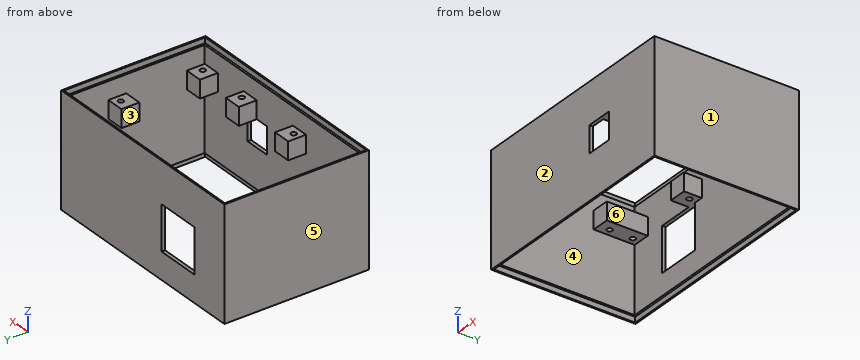
```python
from build123d import *

# Parameters (mm, degrees)
F0_W      = 124.8
F0_H      = 81
F1_DEPTH  = 63
F2_W      = 123.1
F2_H      = 79.3
F3_DEPTH  = 3
F4_W      = 123.1
F4_H      = 79.3
F5_DEPTH  = 3
F6_W      = 120.8
F6_H      = 77
F7_DEPTH  = 60.001
F8_W      = 21
F8_H      = 10
F9_DEPTH  = 10
F10_W     = 23
F10_H     = 10
F11_DEPTH = 10
F12_W     = 10
F12_H     = 10
F13_DEPTH = 10
F14_W     = 10
F14_H     = 10
F15_DEPTH = 10
F16_W     = 10
F16_H     = 10
F17_DEPTH = 10
F18_W     = 10
F18_H     = 10
F19_DEPTH = 10
F20_W     = 10
F20_H     = 10
F21_DEPTH = 10
F22_R     = 1.5
F23_DEPTH = 50.001
F24_R     = 1.5
F25_DEPTH = 50.001
F26_R     = 1.5
F27_DEPTH = 50.001
F28_R     = 1.5
F29_DEPTH = 50.001
F30_R     = 1.5
F31_DEPTH = 50.001
F32_R     = 1.5
F33_DEPTH = 50.001
F34_R     = 1.5
F35_DEPTH = 50.001
F36_R     = 1.5
F37_DEPTH = 50.001
F38_R     = 1.5
F39_DEPTH = 50.001
F40_W     = 25
F40_H     = 25
F41_DEPTH = 2.001
F42_W     = 15
F42_H     = 15
F43_DEPTH = 12


with BuildPart() as f1:
    # F0 (on Top) → F1 (new body)
    with BuildSketch(Plane.XY):
        Rectangle(F0_W, F0_H)
    extrude(amount=F1_DEPTH)

    # F2 (on face) → F3 (cut)
    with BuildSketch(Plane(origin=(0, 0, 0), x_dir=(1, 0, 0), z_dir=(0, 0, -1))):
        Rectangle(F2_W, F2_H)
    extrude(amount=-F3_DEPTH, mode=Mode.SUBTRACT)

    # F4 (on face) → F5 (cut)
    with BuildSketch(Plane.XY.offset(63)):
        Rectangle(F4_W, F4_H)
    extrude(amount=-F5_DEPTH, mode=Mode.SUBTRACT)

    # F6 (on face) → F7 (cut, through all)
    with BuildSketch(Plane.XY.offset(60)):
        Rectangle(F6_W, F6_H)
    extrude(amount=-F7_DEPTH, mode=Mode.SUBTRACT)

    # F8 (on face) → F9 (join)
    with BuildSketch(Plane.YZ.offset(-60.4)):
        with Locations((-28, 45)):
            Rectangle(F8_W, F8_H)
    extrude(amount=F9_DEPTH)

    # F10 (on face) → F11 (join)
    with BuildSketch(Plane.YZ.offset(-60.4)):
        with Locations((27, 45)):
            Rectangle(F10_W, F10_H)
    extrude(amount=F11_DEPTH)

    # F12 (on face) → F13 (join)
    with BuildSketch(Plane(origin=(60.4, 0, 0), x_dir=(0, -1, 0), z_dir=(-1, 0, 0))):
        with Locations((33.5, 45)):
            Rectangle(F12_W, F12_H)
    extrude(amount=F13_DEPTH)

    # F14 (on face) → F15 (join)
    with BuildSketch(Plane(origin=(60.4, 0, 0), x_dir=(0, -1, 0), z_dir=(-1, 0, 0))):
        with Locations((-10.5, 45)):
            Rectangle(F14_W, F14_H)
    extrude(amount=F15_DEPTH)

    # F16 (on face) → F17 (join)
    with BuildSketch(Plane(origin=(0, -38.5, 0), x_dir=(-1, 0, 0), z_dir=(0, 1, 0))):
        with Locations((-25.6, 45)):
            Rectangle(F16_W, F16_H)
    extrude(amount=F17_DEPTH)

    # F18 (on face) → F19 (join)
    with BuildSketch(Plane(origin=(0, -38.5, 0), x_dir=(-1, 0, 0), z_dir=(0, 1, 0))):
        with Locations((12.1, 45)):
            Rectangle(F18_W, F18_H)
    extrude(amount=F19_DEPTH)

    # F20 (on face) → F21 (join)
    with BuildSketch(Plane.XZ.offset(-38.5)):
        with Locations((-14.06, 45)):
            Rectangle(F20_W, F20_H)
    extrude(amount=F21_DEPTH)

    # F22 (on face) → F23 (cut, through all)
    with BuildSketch(Plane.XY.offset(50)):
        with Locations((-56.4, -34.5)):
            Circle(F22_R)
    extrude(amount=-F23_DEPTH, mode=Mode.SUBTRACT)

    # F24 (on face) → F25 (cut, through all)
    with BuildSketch(Plane.XY.offset(50)):
        with Locations((-56.4, -23.5)):
            Circle(F24_R)
    extrude(amount=-F25_DEPTH, mode=Mode.SUBTRACT)

    # F26 (on face) → F27 (cut, through all)
    with BuildSketch(Plane.XY.offset(50)):
        with Locations((-56.4, 34.5)):
            Circle(F26_R)
    extrude(amount=-F27_DEPTH, mode=Mode.SUBTRACT)

    # F28 (on face) → F29 (cut, through all)
    with BuildSketch(Plane.XY.offset(50)):
        with Locations((-56.4, 21.5)):
            Circle(F28_R)
    extrude(amount=-F29_DEPTH, mode=Mode.SUBTRACT)

    # F30 (on face) → F31 (cut, through all)
    with BuildSketch(Plane.XY.offset(50)):
        with Locations((56.4, -34.5)):
            Circle(F30_R)
    extrude(amount=-F31_DEPTH, mode=Mode.SUBTRACT)

    # F32 (on face) → F33 (cut, through all)
    with BuildSketch(Plane.XY.offset(50)):
        with Locations((56.4, 11.5)):
            Circle(F32_R)
    extrude(amount=-F33_DEPTH, mode=Mode.SUBTRACT)

    # F34 (on face) → F35 (cut, through all)
    with BuildSketch(Plane.XY.offset(50)):
        with Locations((26.6, -34.5)):
            Circle(F34_R)
    extrude(amount=-F35_DEPTH, mode=Mode.SUBTRACT)

    # F36 (on face) → F37 (cut, through all)
    with BuildSketch(Plane.XY.offset(50)):
        with Locations((-13.1, -34.5)):
            Circle(F36_R)
    extrude(amount=-F37_DEPTH, mode=Mode.SUBTRACT)

    # F38 (on face) → F39 (cut, through all)
    with BuildSketch(Plane.XY.offset(50)):
        with Locations((-13.06, 34.5)):
            Circle(F38_R)
    extrude(amount=-F39_DEPTH, mode=Mode.SUBTRACT)

    # F40 (on face) → F41 (cut, through all)
    with BuildSketch(Plane.XZ.offset(-38.5)):
        with Locations((-26.9, 27.5)):
            Rectangle(F40_W, F40_H)
    extrude(amount=-F41_DEPTH, mode=Mode.SUBTRACT)

    # F42 (on face) → F43 (cut)
    with BuildSketch(Plane.XZ.offset(40.5)):
        with Locations((20.1, 32.5)):
            Rectangle(F42_W, F42_H)
    extrude(amount=-F43_DEPTH, mode=Mode.SUBTRACT)


solid = f1.part
```
Work out the finished part from the listing and answer in its coordinate system (mm). Face numbers are marked on the shaded views. A direction names the side the tool comes from. Give positions to 0.01 mm unless a question says otherwise; leave off trailing zeros. Loops run counter-clockwise (first coordinate to the right, second up) from the corner with the lowest first, then second, coordinate; pieces in that order, holes last. Notation, with made-up numbers: M 43.5,56 L 85.5,56 A19 ccw 85.5,74 Z; hole C 66,84 d7. An arc over 180 degrees is marked long. One line per item, written item: value. Start each with the question number.
1. Determine the mould class of the marked faces 1, 2 and 3 for opening direction Y: released by +Y, released by -Y, zero draft, split by the parting line, or undercut.
2. Find section D-D (x = 11). Give the vertices of the cut face in (y, z).
3. Which of the six approach directions +Z, -Z, +X, -X, +Y, -Y give full straight-line access (tool end or side, diameter ignored) to the marked faces 4, 5 and 6?
4. Find section C-C (x = -30). Give the vertices of the cut face in (y, z).
5. Each of these flat-tipped pins is pushed along its axis until it touches: P1, Ø10, axis at x = 25.5, y = -29, coming from the +Z side; P2, Ø4, axis at x = 56.4, y = -34.5, coming from the -Z side. Where does it stop, or does it pass through?
6. Find section B-B (z = 33.5). Give the vertices of the cut face in (x, y), and give its area (3 significant figures).
7. Find section A-A (y = -23.5). Give the vertices of the cut face in (x, z).
8. Find the intervals of material crossed by probe 1 along Y at (x, z) = (56.4, 45.5); probe 2 along Y at (x, z) = (-56.4, 42.75); probe 3 along Y at (x, z) = (-13.06, 43.75), in increasing order.
Reported:
1. face 1: zero draft
1. face 2: released by -Y
1. face 3: undercut
2. outline: M -40.5,0 L -39.65,0 L -39.65,3 L -38.5,3 L -38.5,60 L -39.65,60 L -39.65,63 L -40.5,63 Z; M 38.5,3 L 39.65,3 L 39.65,0 L 40.5,0 L 40.5,63 L 39.65,63 L 39.65,60 L 38.5,60 Z
3. face 4: none
3. face 5: +Z, -Z, -X, +Y, -Y
3. face 6: +Z, -Z
4. outline: M -40.5,0 L -39.65,0 L -39.65,3 L -38.5,3 L -38.5,60 L -39.65,60 L -39.65,63 L -40.5,63 Z; M 38.5,3 L 39.65,3 L 39.65,0 L 40.5,0 L 40.5,15 L 38.5,15 Z; M 38.5,40 L 40.5,40 L 40.5,63 L 39.65,63 L 39.65,60 L 38.5,60 Z
5. P1: stops at z = 50
5. P2: stops at z = 40
6. outline: M -62.4,-40.5 L 12.6,-40.5 L 12.6,-38.5 L -60.4,-38.5 L -60.4,38.5 L -39.4,38.5 L -39.4,40.5 L -62.4,40.5 Z; M -14.4,38.5 L 60.4,38.5 L 60.4,-38.5 L 27.6,-38.5 L 27.6,-40.5 L 62.4,-40.5 L 62.4,40.5 L -14.4,40.5 Z
6. area: 727 mm²
7. outline: M -62.4,0 L -61.55,0 L -61.55,3 L -60.4,3 L -60.4,40 L -57.9,40 L -57.9,50 L -60.4,50 L -60.4,60 L -61.55,60 L -61.55,63 L -62.4,63 Z; M -54.9,40 L -50.4,40 L -50.4,50 L -54.9,50 Z; M 60.4,3 L 61.55,3 L 61.55,0 L 62.4,0 L 62.4,63 L 61.55,63 L 61.55,60 L 60.4,60 Z
8. probe 1: y = -40.5 to -36, -33 to -28.5, 5.5 to 10, 13 to 15.5, 38.5 to 40.5
8. probe 2: y = -40.5 to -36, -33 to -25, -22 to -17.5, 15.5 to 20, 23 to 33, 36 to 40.5
8. probe 3: y = -40.5 to -36, -33 to -28.5, 28.5 to 33, 36 to 40.5
